from build123d import *

# Parameters (mm, degrees)
CROQUIS1_R              = 18
SALIENTE_EXTRUIR1_DEPTH = 29
CROQUIS2_R              = 2.5
SALIENTE_EXTRUIR2_DEPTH = 22
CROQUIS3_R              = 18
CROQUIS3_R_2            = 5
CORTAR_EXTRUIR1_DEPTH   = 1


with BuildPart() as part:
    # Croquis1 → Saliente-Extruir1 (new body)
    with BuildSketch(Plane(origin=(0, 0, 0), x_dir=(1, 0, 0), z_dir=(0, 1, 0))):
        Circle(CROQUIS1_R)
    extrude(amount=SALIENTE_EXTRUIR1_DEPTH)

    # Croquis2 → Saliente-Extruir2 (add)
    with BuildSketch(Plane.XZ):
        Circle(CROQUIS2_R)
    extrude(amount=SALIENTE_EXTRUIR2_DEPTH)

    # Croquis3 → Cortar-Extruir1 (cut)
    with BuildSketch(Plane(origin=(0, 29, 0), x_dir=(1, 0, 0), z_dir=(0, 1, 0))):
        Circle(CROQUIS3_R)
        Circle(CROQUIS3_R_2, mode=Mode.SUBTRACT)
    extrude(amount=-CORTAR_EXTRUIR1_DEPTH, mode=Mode.SUBTRACT)

    # Croquis4 → Cortar-Revolución1 (revolve, cut)
    with BuildSketch(Plane.XY):
        Polygon((-18, 22.5), (-11.25, 28), (-18, 28), align=None)
    revolve(axis=Axis((0, 0, 0), (0, 1, 0)), mode=Mode.SUBTRACT)


solid = part.part
Check sheet for the modelled part. Datum: model origin and axes. Units: mm. A direction names the side the tool comes from. Give positions to 0.01 mm unless a question says otherwise; leave off trailing zeros. Loops run counter-clockwise (first coordinate to the right, second up) from the corner with the lowest first, then second, coordinate; pieces in that order, holes last. Notation, with made-up numbers: M -22,73 L 37,73 A28 ccw 37,107 Z; hole C -1,66 d5. An arc over 180 degrees is marked long. Return JSON: item names as keys, results as strings. Group by question number.
1. Tool access check on faces 1 (the cylindrical face through (-2.343, 11.092, -17.847)), 2 (the cylindrical face through (-1.08, 28.51, 4.88)), 3 (the cylindrical face through (-0.54, -10.85, -2.44)). Record the directions out of +Z, -Z, +X, -X, +Y, -Y that give a thin tool (end or side, any length) a straight path to the whole face; none if there is none.
2. Thickness scan on L1, parallel to X at y = 13, z = -0.5; L2, parallel to Y at x = -3.5, z = 3; L3, parallel to Y at x = 1, z = 8. Record the ranges inside material, lowest first.
3. Cross-section at C-C on y = -8.5. Record the boundary of the cut face in (x, z).
4. Cross-section at D-D on y = 17. Record the boundary of the cut face in (x, z), plus the area to 3 significant figures.
5. Go/stop test with flat-tipped pins: pin 1 (1.5 mm diameter, centred on x = 5.5, z = -12, fed in from +Y); pin 2 (2 mm diameter, centred on x = -2, z = 13, fed in from -Y); pin 3 (2 mm diameter, centred on y = 17.5, z = -3.5, fed in from -X). Record where each tip stops, or that it passes through.
6. Cross-section at A-A on x = 0. Record the boundary of the cut face in (y, z), plus the area to 3 significant figures.
7. Cross-section at B-B on z = 0. Record the boundary of the cut face in (x, y), plus the area to 3 significant figures.
Return value:
{
 "1": {"face 1": "+Y, -Y", "face 2": "+Y", "face 3": "-Y"},
 "2": {"L1": "-17.99 to 17.99", "L2": "0 to 29", "L3": "0 to 28"},
 "3": {"outline": "C 0,0 d5"},
 "4": {"outline": "C 0,0 d36", "area": "1,020 mm^2"},
 "5": {"pin 1": "y = 27.02", "pin 2": "y = 0", "pin 3": "x = -17.83"},
 "6": {"outline": "M -22,-2.5 L 0,-2.5 L 0,-18 L 22.5,-18 L 28,-11.25 L 28,-5 L 29,-5 L 29,5 L 28,5 L 28,11.25 L 22.5,18 L 0,18 L 0,2.5 L -22,2.5 Z", "area": "1,090 mm^2"},
 "7": {"outline": "M -18,0 L -2.5,0 L -2.5,-22 L 2.5,-22 L 2.5,0 L 18,0 L 18,22.5 L 11.25,28 L 5,28 L 5,29 L -5,29 L -5,28 L -11.25,28 L -18,22.5 Z", "area": "1,090 mm^2"}
}
